Autodesk Inventor part; units mm, degrees
ref_plane "YZ Plane" through (0, 0, 0) normal (1, 0, 0) x (0, 1, 0)
ref_plane "XZ Plane" through (0, 0, 0) normal (0, 1, 0) x (-1, 0, 0)
ref_plane "XY Plane" through (0, 0, 0) normal (0, 0, 1) x (1, 0, 0)
sketch "Sketch1" plane through (0, 0, 0) normal (0, 0, 1) x (1, 0, 0)
  line L0 (-62, 19) -> (62, 19)
  line L1 (70, 11) -> (70, -11)
  line L2 (62, -19) -> (-62, -19)
  line L3 (-70, -11) -> (-70, 11)
  arc A0 (-62, 19) -> (-70, 11) centre (-62, 11) ccw
  arc A1 (-70, -11) -> (-62, -19) centre (-62, -11) ccw
  arc A2 (70, 11) -> (62, 19) centre (62, 11) ccw
  arc A3 (62, -19) -> (70, -11) centre (62, -11) ccw
  point P0 (0, 0)
  point P1 (70, -19)
  point P2 (70, 19)
  point P3 (-70, -19)
  dimension "d0" = 140
  dimension "d1" = 38
  dimension "d2" = 70
  dimension "d3" = 19
  dimension "d4" = 8
  dimension "d5" = 8
  dimension "d6" = 8
  dimension "d7" = 8
extrude "Extrusion1" add sketch "Sketch1" against normal blind 18
sketch "Sketch2" plane through (0, 0, 0) normal (0, 0, 1) x (1, 0, 0)
  line L0 (-62, 19) -> (62, 19)
  arc A0 (-62, 19) -> (-70, 11) centre (-62, 11) ccw
  line L1 (-70, -11) -> (-70, 11)
  arc A1 (-70, -11) -> (-62, -19) centre (-62, -11) ccw
  line L2 (62, -19) -> (-62, -19)
  arc A2 (62, -19) -> (70, -11) centre (62, -11) ccw
  line L3 (70, 11) -> (70, -11)
  arc A3 (70, 11) -> (62, 19) centre (62, 11) ccw
  line L4 (62, 17) -> (-62, 17)
  arc A4 (-62, 17) -> (-68, 11) centre (-62, 11) ccw
  line L5 (-68, 11) -> (-68, -11)
  arc A5 (-68, -11) -> (-62, -17) centre (-62, -11) ccw
  line L6 (-62, -17) -> (62, -17)
  arc A6 (62, -17) -> (68, -11) centre (62, -11) ccw
  line L7 (68, -11) -> (68, 11)
  arc A7 (68, 11) -> (62, 17) centre (62, 11) ccw
  point P0 (0, 0)
  dimension "d10" = 2
extrude "Extrusion2" cut sketch "Sketch2" against normal blind 14 contours A7 L7 A6 L6 A5 L5 A4 L4
sketch "Sketch3" plane through (70, -11, 0) normal (1, 0, 0) x (0, 0, -1)
  line L0 (0, 22) -> (0, 0)
  line L1 (-6.9158, 18.5) -> (10, 18.5)
  line L2 (10, 18.5) -> (10, 3.5)
  line L3 (10, 3.5) -> (-6.9158, 3.5)
  line L4 (-6.9158, 3.5) -> (-6.9158, 18.5)
  point P0 (0, 11)
  dimension "d13" = 6.9158
  dimension "d14" = 10
  dimension "d15" = 15
  dimension "d16" = 7.5
extrude "Extrusion3" cut sketch "Sketch3" against normal blind 14
sketch "Sketch4" plane through (0, 0, -14) normal (0, 0, 1) x (1, 0, 0)
  line L0 (-62, -17) -> (62, -17)
  line L1 (62, 17) -> (-62, 17)
  line L2 (27, 19) -> (32, 19)
  line L3 (32, 19) -> (32, 16)
  line L4 (32, 16) -> (27, 16)
  line L5 (27, 16) -> (27, 19)
  line L6 (32, -19) -> (27, -19)
  line L7 (27, -19) -> (27, -16)
  line L8 (27, -16) -> (32, -16)
  line L9 (32, -16) -> (32, -19)
  line L10 (-42, -19) -> (-47, -19)
  line L11 (-47, -19) -> (-47, -16)
  line L12 (-47, -16) -> (-42, -16)
  line L13 (-42, -16) -> (-42, -19)
  line L14 (70, 7.5) -> (70, -7.5)
  line L15 (62, -19) -> (-62, -19)
  line L16 (-62, 19) -> (62, 19)
  line L17 (-39, 19) -> (-34, 19)
  line L18 (-34, 19) -> (-34, 16)
  line L19 (-34, 16) -> (-39, 16)
  line L20 (-39, 16) -> (-39, 19)
  line L21 (-70, -11) -> (-70, 11)
  point P0 (0, 0)
  dimension "d19" = 38
  dimension "d20" = 5
  dimension "d21" = 5
  dimension "d22" = 38
  dimension "d23" = 1
  dimension "d24" = 1
  dimension "d25" = 0
  dimension "d26" = 0
  dimension "d28" = 1
  dimension "d29" = 0
  dimension "d30" = 5
  dimension "d31" = 5
  dimension "d33" = 1
  dimension "d34" = 0
  dimension "d59" = 66
  dimension "d60" = 74
extrude "Extrusion4" add sketch "Sketch4" along normal blind 13 contours L11 L12 L13 L0 | L0 L13 L10 L11 | L7 L8 L9 L0 | L0 L9 L6 L7 | L3 L4 L5 L1 | L1 L5 L2 L3 | L18 L19 L20 L1 | L1 L20 L16 L18
chamfer "Chamfer1" distance 1 distance2 1 1 edges at (-36.5, 16, -1) measured on face at (-35.6667, 16, -9.6667)
chamfer "Chamfer3" distance 1 distance2 1 1 edges at (29.5, 16, -1) measured on face at (30.3333, 16, -9.6667)
chamfer "Chamfer4" distance 1 distance2 1 1 edges at (-44.5, -16, -1) measured on face at (-45.3333, -16, -9.6667)
chamfer "Chamfer5" distance 1 distance2 1 1 edges at (29.5, -16, -1) measured on face at (28.6667, -16, -9.6667)
sketch "Sketch5" plane through (0, 0, -14) normal (0, 0, 1) x (1, 0, 0)
  line L0 (-39, 17) -> (-62, 17)
  arc A0 (-62, 17) -> (-68, 11) centre (-62, 11) ccw
  line L1 (-68, 11) -> (-68, -11)
  arc A1 (-68, -11) -> (-62, -17) centre (-62, -11) ccw
  line L2 (-62, -17) -> (-47, -17)
  line L3 (-47, -17) -> (-47, -16)
  line L4 (-47, -16) -> (-42, -16)
  line L5 (-42, -16) -> (-42, -17)
  line L6 (-42, -17) -> (27, -17)
  line L7 (27, -17) -> (27, -16)
  line L8 (27, -16) -> (32, -16)
  line L9 (32, -16) -> (32, -17)
  line L10 (32, -17) -> (62, -17)
  line L11 (-49, 17) -> (37, 17)
  line L12 (37, 17) -> (37, -17)
  line L13 (37, -17) -> (-49, -17)
  line L14 (-49, -17) -> (-49, 17)
  point P0 (32, 16)
  point P1 (-39, 16)
  point P2 (0, 0)
  dimension "d53" = 10
  dimension "d54" = 5
extrude "Extrusion5" cut sketch "Sketch5" along normal blind 11
sketch "Sketch6" plane through (0, 0, -14) normal (0, 0, 1) x (1, 0, 0)
  arc A0 (62, -17) -> (68, -11) centre (62, -11) ccw
  arc A1 (-62, 17) -> (-68, 11) centre (-62, 11) ccw
  line L0 (-62, 11) -> (62, 11)
  line L1 (62, 11) -> (62, -11)
  line L2 (62, -11) -> (-62, -11)
  line L3 (-62, -11) -> (-62, 11)
  point P0 (0, 0)
extrude "Extrusion6" cut sketch "Sketch6" against normal through all
sketch "Sketch8" plane through (0, 0, 0) normal (0, 0, 1) x (1, 0, 0)
  line L0 (-70, -11) -> (-70, 11)
  line L1 (62, -19) -> (-62, -19)
  line L2 (70, -7.5) -> (70, -11)
  line L3 (62, -17) -> (-62, -17)
  line L4 (0, -22.5) -> (0, -17) construction
  arc A0 (-52, -18.8579) -> (52, -18.8579) centre (0, 350.5357) ccw
  arc A1 (-49.9899, -19.1353) -> (-52, -19) centre (-52, -34) ccw
  arc A2 (52, -19) -> (49.9899, -19.1353) centre (52, -34) ccw
  line L5 (-52, -19) -> (-52, -17)
  line L6 (52, -19) -> (52, -17)
  line L7 (52, -17) -> (-52, -17)
  point P0 (0, 0)
  dimension "d63" = 2
  dimension "d64" = 18
  dimension "d65" = 18
  dimension "d66" = 5.5
  dimension "d67" = 30
  dimension "d68" = 30
extrude "Extrusion8" add sketch "Sketch8" against normal up to surface (18 mm away) contours A0 L1 | L1 A0 L5 L3 L6
sketch "Sketch9" plane through (0, 0, -18) normal (0, 0, -1) x (-1, 0, 0)
  line L0 (70, 11) -> (70, -11)
  line L1 (62, 11) -> (62, -11)
  line L2 (62, -11) -> (-62, -11)
  line L3 (58, -4) -> (74, -4)
  line L4 (74, -4) -> (74, -8)
  line L5 (74, -8) -> (58, -8)
  line L6 (58, -8) -> (58, -4)
  point P0 (0, 0)
  dimension "d71" = 3
  dimension "d72" = 4
  dimension "d73" = 4
  dimension "d74" = 4
extrude "Extrusion9" cut sketch "Sketch9" against normal blind 10
fillet "Fillet1" radius 2 2 edges at (-69, -8, -8) (-69, -4, -8)
sketch "Sketch10" plane through (0, 0, -14) normal (0, 0, 1) x (1, 0, 0)
  line L0 (-62, -8) -> (-68, -8)
  line L1 (-68, -8) -> (-68, -11)
  arc A0 (-68, -11) -> (-62, -17) centre (-62, -11) ccw
  line L2 (-62, -17) -> (62, -17)
  arc A1 (62, -17) -> (68, -11) centre (62, -11) ccw
  line L3 (68, -11) -> (68, 11)
  arc A2 (68, 11) -> (62, 17) centre (62, 11) ccw
  line L4 (62, 17) -> (-62, 17)
  arc A3 (-62, 17) -> (-68, 11) centre (-62, 11) ccw
  line L5 (-68, 11) -> (-68, -4)
  line L6 (-68, -4) -> (-62, -4)
  line L7 (-62, -4) -> (-62, 11)
  line L8 (-62, 11) -> (62, 11)
  line L9 (62, 11) -> (62, -11)
  line L10 (62, -11) -> (-62, -11)
  line L11 (-62, -11) -> (-62, -8)
  point P0 (0, 0)
properties part number "mainmount"
For this review, take the finished solid that the model builds, in its own axes (mm). A direction names the side the tool comes from. Give positions to 0.01 mm unless a question says otherwise; leave off trailing zeros. Loops run counter-clockwise (first coordinate to the right, second up) from the corner with the lowest first, then second, coordinate; pieces in that order, holes last. Notation, with made-up numbers: (30.5, -36.5) - (89.5, -36.5) arc R34 ccw to (89.5, 1.5) - close; hole circle Ø10 at (78.5, 79.5). An arc over 180 degrees is marked (long way). Write each question's results on one line, items separated by ' | '.
(1) Take a section at B-B (y = -9.5). Give the boundary of the cut face in (x, z), then the cut area to 3 significant figures.
Conclusion:
outline: (-70, -18) - (-62, -18) - (-62, -14) - (-68, -14) - (-68, 0) - (-70, 0) - close; (62, -18) - (70, -18) - (70, 0) - (68, 0) - (68, -14) - (62, -14) - close | area: 120 mm^2
(2) For pin 1 Ø4.5 at (x, z) = (13, -16) entering from -Y; pin 2 Ø3 at (x, z) = (5, -11) entering from -Y; pin 3 Ø1.1 at (y, z) = (-16.5, -2) entering from +X; pin 4 Ø6 at (x, y) = (4, 6.5) entering from +Z, all flat-tipped, find the tip position at first contact; note any pin that passes through.
Conclusion:
pin 1: y = -22.35 | pin 2: y = -22.48 | pin 3: x = 68.28 | pin 4: through
(3) Take a section at A-A (x = -54). Give the boundary of the cut face in (y, z), then the cut area to 3 significant figures.
Conclusion:
outline: (-19, -18) - (-11, -18) - (-11, -14) - (-17, -14) - (-17, 0) - (-19, 0) - close; (11, -18) - (19, -18) - (19, 0) - (17, 0) - (17, -14) - (11, -14) - close | area: 120 mm^2
(4) For faces 5 (the flat face through (-67, -4, -15)), 6 (the cylindrical face through (66.196, -15.289, -6.902)), 7 (the flat face through (57, -19, -9)), 8 (the flat face through (-1, 11, -16)), list the 3-axis set-ups (+Z, -Z, +X, -X, +Y, -Y) from which the entire face can be reached by the end or side of a thin tool; tool diameter is ignored.
Conclusion:
face 5: -Z, -X | face 6: +Z | face 7: +Z, -Z, +X, -Y | face 8: +Z, -Z
(5) For line 1 along Y through (x, z) = (2.5, -15.5); line 2 along X through (y, z) = (4, -11.75); line 3 along Y through (x, z) = (-61, -5.5), list the stretches that pass through material, from the lowest coordinate up.
Conclusion:
line 1: -22.49 to -11, 11 to 19 | line 2: -70 to -68, 68 to 70 | line 3: -19 to -17, 17 to 19
(6) Take a section at C-C (z = -5.25). Give the boundary of the cut face in (x, y), then the cut area to 3 significant figures.
Conclusion:
outline: (-70, -11) arc R8 ccw to (-62, -19) - (-50.98, -19) arc R373.04 ccw to (50.98, -19) - (62, -19) arc R8 ccw to (70, -11) - (70, -7.5) - (68, -7.5) - (68, -11) arc R6 cw to (62, -17) - (-62, -17) arc R6 cw to (-68, -11) - (-68, 11) arc R6 cw to (-62, 17) - (62, 17) arc R6 cw to (68, 11) - (68, 7.5) - (70, 7.5) - (70, 11) arc R8 ccw to (62, 19) - (-62, 19) arc R8 ccw to (-70, 11) - close | area: 880 mm^2
(7) Draft analysis for pull direction Y (two halves, no side actions). For faces 1 (the flat face through (-1, 19, -9)), 2 (the flat face through (-70, 0, -9)), 3 (the flat face through (-1, -17, -7)), 4 (the cylindrical face through (-67.719, -16.594, -8.874)), state which applies: +Y half, -Y half, draft (parallel to the pull), parting line (faces both ways), or undercut.
Conclusion:
face 1: +Y half | face 2: draft | face 3: undercut | face 4: -Y half
